Source: CAD feature listing. Evaluate the final solid. Frame: model axes, mm. Face numbers are marked on the shaded views. Round coordinates to 2 decimals unless told otherwise and drop trailing zeros. Loops run counter-clockwise (first coordinate to the right, second up) from the corner with the lowest first, then second, coordinate; pieces in that order, holes last.
Item 1: Section query C-C on x = -60.5. Return loops of the section in (y, z), then the cut area to 3 significant figures.
Item 2: First-contact query: P1, Ø4, axis at x = -44.5, y = 119.5, coming from the -Z side. Flat tip, straight axial feed; report the tip coordinate or a pass-through.
Item 3: Ray query, L1, parallel to Y at x = -48, z = 3.5; L2, parallel to X at y = 85.5, z = 0.2; L3, parallel to Y at x = -18, z = 0.85. Return the intervals inside material, ascending.
Item 4: Pull-direction query (X, two-part tool) for the marked faces 1, 2 and 3; classes: released by +X, released by -X, zero draft, split by the parting line, or undercut.
Item 5: Section query B-B on y = 85.5. Return loops of the section in (x, z), then the cut area to 3 significant figures.
Item 6: Section query D-D on y = 44. Return loops of the section in (x, z).
Item 7: Section query A-A on z = 4.25. Return loops of the section in (x, y), then the cut area to 3 significant figures.
Autodesk Inventor part; units mm, degrees
ref_plane "YZ Plane" through (0, 0, 0) normal (1, 0, 0) x (0, 1, 0)
ref_plane "XZ Plane" through (0, 0, 0) normal (0, 1, 0) x (-1, 0, 0)
ref_plane "XY Plane" through (0, 0, 0) normal (0, 0, 1) x (1, 0, 0)
sketch "Sketch1" plane through (0, 0, 0) normal (0, 0, 1) x (1, 0, 0)
  line L0 (0, 0) -> (-75, 0)
  line L1 (-75, 0) -> (-75, 180)
  line L2 (-75, 180) -> (0, 180)
  line L3 (0, 180) -> (0, 0)
  line L4 (-65, 170) -> (-10, 170)
  line L5 (-10, 10) -> (-65, 10)
  line L6 (-65, 10) -> (-65, 85)
  line L7 (-65, 95) -> (-65, 170)
  line L8 (-10, 170) -> (-10, 95)
  line L9 (-10, 85) -> (-10, 10)
  line L10 (-65, 85) -> (-65, 95)
  line L11 (-10, 95) -> (-10, 85)
  point P0 (-65, 90)
  point P1 (-10, 90)
  dimension "d35" = 75
  dimension "d36" = 180
  dimension "d37" = 55
  dimension "d38" = 160
extrude "Extrusion16" add sketch "Sketch1" along normal blind 1
sketch "Sketch12" plane through (0, 0, 1) normal (0, 0, 1) x (1, 0, 0)
  line L0 (0, 0) -> (0, 180)
  line L1 (-75, 180) -> (-75, 0)
  line L2 (0, 180) -> (-75, 180)
  line L3 (-75, 180) -> (-75, 0)
  line L4 (-75, 0) -> (0, 0)
  line L5 (0, 0) -> (0, 180)
extrude "Extrusion17" add sketch "Sketch12" along normal blind 4
sketch "Sketch13" plane through (0, 0, 5) normal (0, 0, 1) x (1, 0, 0)
  line L0 (-10, 117.5) -> (-65, 117.5)
  line L1 (-65, 117.5) -> (-65, 62.5)
  line L2 (-65, 62.5) -> (-10, 62.5)
  line L3 (-10, 62.5) -> (-10, 117.5)
  point P0 (0, 0)
  dimension "d99" = 55
  dimension "d100" = 55
extrude "Extrusion18" cut sketch "Sketch13" against normal blind 2
properties part number "Shoulder_Cube_TestFit_V1"
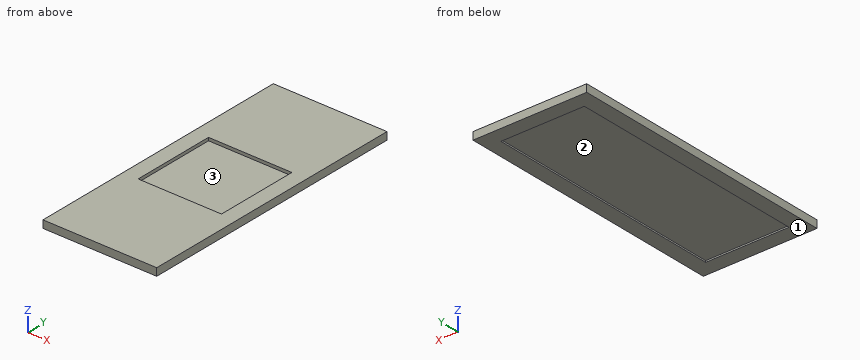
Data:
1. outline: (0, 0) - (10, 0) - (10, 1) - (170, 1) - (170, 0) - (180, 0) - (180, 5) - (117.5, 5) - (117.5, 3) - (62.5, 3) - (62.5, 5) - (0, 5) - close
1. area: 630 mm2
2. P1: stops at z = 1
3. L1: y = 0 to 62.5, 117.5 to 180
3. L2: x = -75 to -65, -10 to 0
3. L3: y = 0 to 10, 170 to 180
4. face 1: zero draft
4. face 2: undercut
4. face 3: undercut
5. outline: (-75, 0) - (-65, 0) - (-65, 1) - (-10, 1) - (-10, 0) - (0, 0) - (0, 5) - (-10, 5) - (-10, 3) - (-65, 3) - (-65, 5) - (-75, 5) - close
5. area: 210 mm2
6. outline: (-75, 0) - (-65, 0) - (-65, 1) - (-10, 1) - (-10, 0) - (0, 0) - (0, 5) - (-75, 5) - close
7. outline: (-75, 0) - (0, 0) - (0, 180) - (-75, 180) - close; hole (-65, 62.5) - (-10, 62.5) - (-10, 117.5) - (-65, 117.5) - close
7. area: 10,500 mm2
